Work out the finished part from the listing and answer in its coordinate system (mm). Round coordinates to 2 decimals unless told otherwise and drop trailing zeros. Order: outer loops, then holes, each group sorted by start corner. A loop starts at its lowest first (then second) coordinate and runs counter-clockwise, first axis right, second up.
from build123d import *

# Parameters (mm, degrees)
EXTRUDE_1_DEPTH     = 3
SKETCH_2_R          = 1.575
SKETCH_2_R_2        = 6.8
CUT_EXTRUDE_2_DEPTH = 65.101482042
FILLET_1_R          = 5


with BuildPart() as part:
    # 草图1 → 凸台-拉伸1 (new body)
    with BuildSketch(Plane.XY):
        Polygon((0, 0), (0, -20), (10, -50), (30, -50), (40, -20), (40, 0), align=None)
    extrude(amount=EXTRUDE_1_DEPTH)

    # 草图2 → 切除-拉伸2 (cut, through all)
    with BuildSketch(Plane.XY.offset(3)):
        with Locations((5, -5)):
            Circle(SKETCH_2_R)
        with Locations(Location((15, -5, 0), (0, 0, 180))):
            Circle(SKETCH_2_R)
        with Locations((15, -15)):
            Circle(SKETCH_2_R)
        with Locations(Location((5, -15, 0), (0, 0, 180))):
            Circle(SKETCH_2_R)
        with Locations((35, -15)):
            Circle(SKETCH_2_R)
        with Locations(Location((25, -15, 0), (0, 0, 180))):
            Circle(SKETCH_2_R)
        with Locations((25, -5)):
            Circle(SKETCH_2_R)
        with Locations(Location((35, -5, 0), (0, 0, 180))):
            Circle(SKETCH_2_R)
        with Locations((20, -35)):
            Circle(SKETCH_2_R_2)
        with Locations((20, -25.5)):
            Circle(SKETCH_2_R)
        with Locations((28.227241336, -39.75)):
            Circle(SKETCH_2_R)
        with Locations((11.772758664, -39.75)):
            Circle(SKETCH_2_R)
    extrude(amount=-CUT_EXTRUDE_2_DEPTH, mode=Mode.SUBTRACT)

    # 圆角1
    fillet_1_edges = [part.edges().sort_by_distance(p)[0] for p in [
        (40, 0, 1.5),
        (40, -20, 1.5),
        (30, -50, 1.5),
        (10, -50, 1.5),
        (0, -20, 1.5),
        (0, 0, 1.5),
    ]]
    fillet(fillet_1_edges, radius=FILLET_1_R)


solid = part.part
Item 1: Find section A-A (y = -35). Write down the section's boundary in (x, z).
Item 2: Find the intervals of material crossed by line 1 along Y through (x, z) = (20, 1.1) (3 decimals); line 2 along X through (y, z) = (-40.5, 2.2); line 3 along X through (y, z) = (-29, 1.15), in increasing order.
Item 3: Find section D-D (z = 0.6). State how many separate pieces and enclosed holes the cut face has, plus the area to 3 significant figures.
Item 4: For a pull along X with two mould halves and no side action, classify faces 1 (the face through (38, -1, 2)), 2 (the face through (20, -19, 3)), 3 (the face through (16.502, -14.527, 1.521)) as released by +X, released by -X, zero draft, split by the parting line, or undercut.
Item 5: Find section B-B (x = 20). Write down the section's boundary in (y, z) (3 decimals).
Item 6: Find section C-C (y = -15). Write down the section's boundary in (x, z) (3 decimals), plus the area to 3 significant figures.
Model answer:
1. outline: (5, 0) - (13.2, 0) - (13.2, 3) - (5, 3) - close; (26.8, 0) - (35, 0) - (35, 3) - (26.8, 3) - close
2. line 1: y = -50 to -41.8, -28.2 to -27.075, -23.925 to 0
2. line 2: x = 6.83 to 10.39, 13.16 to 16, 24 to 26.84, 29.61 to 33.17
2. line 3: x = 3 to 16.8, 23.2 to 37
3. separate pieces: 1
3. enclosed holes: 12
3. area: 1,450 mm2
4. face 1: released by +X
4. face 2: zero draft
4. face 3: undercut
5. outline: (-50, 0) - (-41.8, 0) - (-41.8, 3) - (-50, 3) - close; (-28.2, 0) - (-27.075, 0) - (-27.075, 3) - (-28.2, 3) - close; (-23.925, 0) - (0, 0) - (0, 3) - (-23.925, 3) - close
6. outline: (0, 0) - (3.425, 0) - (3.425, 3) - (0, 3) - close; (6.575, 0) - (13.425, 0) - (13.425, 3) - (6.575, 3) - close; (16.575, 0) - (23.425, 0) - (23.425, 3) - (16.575, 3) - close; (26.575, 0) - (33.425, 0) - (33.425, 3) - (26.575, 3) - close; (36.575, 0) - (40, 0) - (40, 3) - (36.575, 3) - close
6. area: 82.2 mm2
